from build123d import *

# Parameters (mm, degrees)
SKETCH1_R               = 3.175
BOSS_EXTRUDE1_DEPTH     = 35.56
SKETCH3_W               = 0.508
SKETCH3_H               = 0.7366
SKETCH5_R               = 3.175
BOSS_EXTRUDE2_DEPTH     = 25.4
CUT_EXTRUDE1_DEPTH      = 62.1251409
CUT_EXTRUDE1_DEPTH_BACK = 62.1251409
SKETCH4_R               = 0.79375


with BuildPart() as part:
    # Sketch1 → Boss-Extrude1 (new body)
    with BuildSketch(Plane.XY):
        Circle(SKETCH1_R)
    extrude(amount=BOSS_EXTRUDE1_DEPTH)

    # Sketch3 → Cut-Revolve3 (revolve, cut)
    with BuildSketch(Plane(origin=(0, 0, 0), x_dir=(1, 0, 0), z_dir=(0, 1, 0)), mode=Mode.PRIVATE) as cut_revolve3_sk:
        with Locations((2.921, -2.5527)):
            Rectangle(SKETCH3_W, SKETCH3_H)
    revolve(cut_revolve3_sk.sketch.rotate(Axis((0, 0, 0), (0, 0, 1)), 180), axis=Axis((0, 0, 0), (0, 0, 1)), mode=Mode.SUBTRACT)

    # Sketch5 → Boss-Extrude2 (add)
    with BuildSketch(Plane.XY.offset(35.56)):
        with Locations(Location((0, 0, 0), (0, 0, 180))):
            Circle(SKETCH5_R)
    extrude(amount=BOSS_EXTRUDE2_DEPTH)

    # Sketch4 → Cut-Extrude1 (cut, two sides: drawn at the far end of the back side and taken through both)
    with BuildSketch(Plane(origin=(0, 0, 0), x_dir=(1, 0, 0), z_dir=(0, 1, 0)).offset(-CUT_EXTRUDE1_DEPTH_BACK)):
        with Locations(Location((0, -47.244, 0), (0, 0, 270))):
            Circle(SKETCH4_R)
        with Locations(Location((0, -49.53, 0), (0, 0, 270))):
            Circle(SKETCH4_R)
    extrude(amount=CUT_EXTRUDE1_DEPTH + CUT_EXTRUDE1_DEPTH_BACK, mode=Mode.SUBTRACT)


solid = part.part
Can you work these out from the model? Positions are in its coordinate system, mm. A direction names the side the tool comes from. Coordinates: 2 decimals unless noted, no trailing zeros. Loops run counter-clockwise (first coordinate to the right, second up) from the corner with the lowest first, then second, coordinate; pieces in that order, holes last. Notation, with made-up numbers: (23.5, 58) - (39.5, 58) arc R16 cw to (39.5, 88) - close; hole circle Ø2 at (12, -7). An arc over 180 degrees is marked (long way). Put each result on its own line as item: value. Start each with the question number.
Item 1: Suppose I cut it at C-C (z = 47.5). Please give me the cut outline in (x, y) (3 decimals), and give its area (3 significant figures).
Item 2: Suppose I cut it at D-D (z = 26). Please give me the cut outline in (x, y) (3 decimals).
Item 3: For pin 1 (1.5 mm diameter, centred on x = -1.5, z = 6, fed in from +Y); pin 2 (1 mm diameter, centred on y = -1, z = 40, fed in from +X); pin 3 (2 mm diameter, centred on x = -1.5, z = 21, fed in from -Y); pin 4 (1.4 mm diameter, centred on x = 0, z = 47.244, fed in from -Y), each with a flat end and sliding along its axis, tell me the tip position at first contact or that it passes through.
Item 4: If I drill on line 1 along Z through (x, y) = (0, -0.5); line 2 along Z through (x, y) = (2.75, 1.25); line 3 along Z through (x, y) = (-0.5, 1), over which ranges is the centre line in solid material (lowest first)?
Item 5: If we mould it in two halves opening along X, with no side actions, what happens to faces 1 (the face through (0, 0, 60.96)), 2 (the face through (0.03, -0.04, 46.45)), 3 (the face through (0.21, 3.17, 31.53))? For each: +X half, -X half, draft (parallel to the pull), parting line (faces both ways), or undercut.
Item 6: Suppose I cut it at B-B (y = -1.5). Please give me the cut outline in (x, z).
Item 7: Which directions (+Z, -Z, +X, -X, +Y, -Y) give clear straight access to the entire face, cutting with the end or side of a thin tool? Please do faces 4 (the face through (-2, -2, 2.184)), 5 (the face through (-0.69, -3.1, 1.08)).
Here are the results:
1. outline: (-0.751, -3.085) - (-0.751, 3.085) arc R3.175 ccw to start; (0.751, -3.085) arc R3.175 ccw to (0.751, 3.085) - close
1. area: 22.2 mm²
2. outline: circle Ø6.35 at (0, 0)
3. pin 1: y = 3.09
3. pin 2: x = 3.14
3. pin 3: y = -3.14
3. pin 4: through
4. line 1: 0 to 46.45, 48.04 to 48.74, 50.32 to 60.96
4. line 2: 0 to 2.18, 2.92 to 60.96
4. line 3: 0 to 46.63, 47.86 to 48.91, 50.15 to 60.96
5. face 1: draft
5. face 2: undercut
5. face 3: parting line
6. outline: (-2.8, 0) - (2.8, 0) - (2.8, 2.18) - (2.21, 2.18) - (2.21, 2.92) - (2.8, 2.92) - (2.8, 60.96) - (-2.8, 60.96) - (-2.8, 2.92) - (-2.21, 2.92) - (-2.21, 2.18) - (-2.8, 2.18) - close; hole circle Ø1.59 at (0, 47.24); hole circle Ø1.59 at (0, 49.53)
7. face 4: none
7. face 5: +Z, -Z
